Build history of the part. All positions in model axes, mm. A direction names the side the tool comes from. Round coordinates to 2 decimals unless told otherwise and drop trailing zeros. Order: outer loops, then holes, each group sorted by start corner. A loop starts at its lowest first (then second) coordinate and runs counter-clockwise, first axis right, second up. Notation, with made-up numbers: M -24,39.5 L -16,39.5 A17 cw -16,54.5 Z; hole C 25,-31.5 d8. An arc over 180 degrees is marked long. One line per item, written item: value. Start each with the question number.
Item 1: Band-saw the part on B-B, the plane z = 0. Write the cut outline in (x, y).
Item 2: Two-plate mould, pull along Y, no slides. Class faces 1 (the flat face through (0, 51, 0)), 2 (the flat face through (20, 20, -3)), 3 (the flat face through (0, 38, 35.5)), 4 (the flat face through (35.5, 38, 0)): +Y half, -Y half, draft (parallel to the pull), parting line (faces both ways), or undercut.
Item 3: Pin check, flat tips, straight feed: pin 1 (3 mm diameter, centred on x = 0, y = 20.5, fed in from +Z); pin 2 (1.8 mm diameter, centred on y = 12, z = -0.5, fed in from -X); pin 3 (1.8 mm diameter, centred on y = 21, z = 0, fed in from +X). Stop position of each tip, or through.
Item 4: Tool access for faces 5 (the flat face through (3, 20, -20)), 6 (the flat face through (3, 20, 20)), 7 (the cylindrical face through (-15.62, 49.99, -3.47)): list every direction of +Z, -Z, +X, -X, +Y, -Y with a clear straight run to the whole face (end or side of a thin tool).
Item 5: Band-saw the part on A-A, the plane y = 8. Write the cut outline in (x, z), then the cut area to 3 significant figures.
Item 6: Band-saw the part on C-C, the plane x = 0. Write the cut outline in (y, z).
Item 7: Probe L1, parallel to X at y = 3, z = 0; L2, parallel to Z at x = -18, y = 30; L3, parallel to Y at x = -36.5, z = -9. List the from-to ranges inside material, lowest first.
```python
from build123d import *

# Parameters (mm, degrees)
BOSS_EXTRUDE1_DEPTH = 40
CHAMFER1_SIZE       = 4
SKETCH3_R           = 41.5
BOSS_EXTRUDE2_DEPTH = 9
SKETCH4_R           = 16
BOSS_EXTRUDE3_DEPTH = 2
CHAMFER2_SIZE       = 3


with BuildPart() as part:
    # Sketch1 → Boss-Extrude1 (new body)
    with BuildSketch(Plane(origin=(0, 0, 0), x_dir=(1, 0, 0), z_dir=(0, 1, 0))):
        Polygon((3, 3), (37.5, 3), (37.5, -3), (3, -3), (3, -37.5), (-3, -37.5), (-3, -3), (-37.5, -3), (-37.5, 3), (-3, 3), (-3, 37.5), (3, 37.5), align=None)
    extrude(amount=BOSS_EXTRUDE1_DEPTH)

    # Chamfer1
    chamfer1_edges = [part.edges().sort_by_distance(p)[0] for p in [
        (0, 40, -37.5),
        (-37.5, 40, 0),
        (0, 40, 37.5),
        (37.5, 40, 0),
    ]]
    chamfer(chamfer1_edges, length=CHAMFER1_SIZE)

    # Sketch3 → Boss-Extrude2 (add)
    with BuildSketch(Plane(origin=(0, 40, 0), x_dir=(1, 0, 0), z_dir=(0, 1, 0))):
        with Locations(Location((0, 0, 0), (0, 0, 270))):
            Circle(SKETCH3_R)
    extrude(amount=BOSS_EXTRUDE2_DEPTH)

    # Sketch4 → Boss-Extrude3 (add)
    with BuildSketch(Plane(origin=(0, 49, 0), x_dir=(1, 0, 0), z_dir=(0, 1, 0))):
        with Locations(Location((0, 0, 0), (0, 0, 270))):
            Circle(SKETCH4_R)
    extrude(amount=BOSS_EXTRUDE3_DEPTH)

    # Chamfer2
    chamfer2_edges = [part.edges().sort_by_distance(p)[0] for p in [
        (0, 40, -41.5),
    ]]
    chamfer(chamfer2_edges, length=CHAMFER2_SIZE)


solid = part.part
```
Output:
1. outline: M -41.5,43 L -38.5,40 L -33.5,40 L -37.5,36 L -37.5,0 L 37.5,0 L 37.5,36 L 33.5,40 L 38.5,40 L 41.5,43 L 41.5,49 L 16,49 L 16,51 L -16,51 L -16,49 L -41.5,49 Z
2. face 1: +Y half
2. face 2: draft
2. face 3: undercut
2. face 4: undercut
3. pin 1: stops at z = 37.5
3. pin 2: stops at x = -37.5
3. pin 3: stops at x = 37.5
4. face 5: -Z, +X, -Y
4. face 6: +Z, +X, -Y
4. face 7: +Y
5. outline: M -37.5,-3 L -3,-3 L -3,-37.5 L 3,-37.5 L 3,-3 L 37.5,-3 L 37.5,3 L 3,3 L 3,37.5 L -3,37.5 L -3,3 L -37.5,3 Z
5. area: 864 mm²
6. outline: M 0,-37.5 L 36,-37.5 L 40,-33.5 L 40,-38.5 L 43,-41.5 L 49,-41.5 L 49,-16 L 51,-16 L 51,16 L 49,16 L 49,41.5 L 43,41.5 L 40,38.5 L 40,33.5 L 36,37.5 L 0,37.5 Z
7. L1: x = -37.5 to 37.5
7. L2: z = -3 to 3
7. L3: y = 40 to 49
